For this review, take the finished solid that the model builds, in its own axes (mm). Face numbers are marked on the shaded views. A direction names the side the tool comes from. Round coordinates to 2 decimals unless told otherwise and drop trailing zeros. Write each loop counter-clockwise with the first axis right and the second up, starting at its lowest first coordinate (ties: lowest second). Pieces come first, ordered by that corner, then holes.
from build123d import *

# Parameters (mm, degrees)
F0_W      = 25.4
F0_H      = 69.85
F1_DEPTH  = 12.7
F3_DEPTH  = 12.701
F5_DEPTH  = 19.05
F6_R      = 6.5291939121
F7_DEPTH  = 31.751
F8_W      = 50.8
F8_H      = 31.75
F9_DEPTH  = 6.35
F10_R     = 4.3841328913
F10_R_2   = 4.0648477918
F11_DEPTH = 25.4
F13_DEPTH = 141
F14_R     = 5.08
F15_W     = 12.5349015713
F15_H     = 9.3853002578
F16_DEPTH = 12.7
F18_DEPTH = 25.4
F20_DEPTH = 12.7
F22_DEPTH = 25.4
F24_DEPTH = 25.4


# Not quite as in the source:
# - an extrude ends at something that could not be found from the text; its depth is read off the source's solid
# - a feature names something its author has since deleted; it is built from what else it names


with BuildPart() as f1:
    # F0 (on Front) → F1 (new body)
    with BuildSketch(Plane.XZ):
        with Locations((-34.1177975344, 34.925)):
            Rectangle(F0_W, F0_H)
    extrude(amount=F1_DEPTH)

    # F2 (on face) → F3 (cut, through all)
    with BuildSketch(Plane.XZ.offset(12.7)):
        with BuildLine():
            ThreePointArc((-46.8177975344, 57.1627020836), (-34.8779343498, 69.8199859011), (-21.4177975344, 58.7931149299))
            Line((-21.4177975344, 58.7931149299), (-21.4177975344, 69.85))
            Line((-21.4177975344, 69.85), (-46.8177975344, 69.85))
            Line((-46.8177975344, 69.85), (-46.8177975344, 57.1627020836))
        make_face()
    extrude(amount=-F3_DEPTH, mode=Mode.SUBTRACT)

    # F4 (on face) → F5 (join)
    with BuildSketch(Plane.XZ.offset(12.7)):
        with BuildLine():
            Line((-46.8177975344, 57.1627020836), (-46.8177975344, 54.9187152869))
            ThreePointArc((-46.8177975344, 54.9187152869), (-34.3603071914, 44.1520357407), (-21.4177975344, 54.3305374906))
            Line((-21.4177975344, 54.3305374906), (-21.4177975344, 58.7931149299))
            ThreePointArc((-21.4177975344, 58.7931149299), (-34.8779343498, 69.8199859011), (-46.8177975344, 57.1627020836))
        make_face()
        with BuildLine():
            ThreePointArc((-21.4177975344, 54.3305374906), (-21.194958074, 55.7017298658), (-21.1203918045, 57.0889089552))
            ThreePointArc((-21.1203918045, 57.0889089552), (-35.1496925912, 69.9833496353), (-46.8177975344, 54.9187152869))
            Line((-46.8177975344, 54.9187152869), (-46.8177975344, 57.1627020836))
            ThreePointArc((-46.8177975344, 57.1627020836), (-34.8779343498, 69.8199859011), (-21.4177975344, 58.7931149299))
            Line((-21.4177975344, 58.7931149299), (-21.4177975344, 54.3305374906))
        make_face()
    extrude(amount=F5_DEPTH)

    # F6 (on face) → F7 (cut, through all)
    with BuildSketch(Plane.XZ.offset(31.75)):
        with Locations((-34.0607331136, 57.0889089552)):
            Circle(F6_R)
    extrude(amount=-F7_DEPTH, mode=Mode.SUBTRACT)

    # F8 (on Top) → F9 (join)
    with BuildSketch(Plane.XY):
        with Locations((-35.2321754485, -16.0400984287)):
            Rectangle(F8_W, F8_H)
    extrude(amount=F9_DEPTH)

    # F10 (on face) → F11 (cut)
    with BuildSketch(Plane.XY.offset(6.35)):
        with Locations((-52.9474318027, -24.9871537089)):
            Circle(F10_R)
        with Locations((-18.3323584497, -24.9871537089)):
            Circle(F10_R_2)
    extrude(amount=-F11_DEPTH, mode=Mode.SUBTRACT)

    # F12 (on Front) → F13 (cut, through all)
    with BuildSketch(Plane.XZ):
        with BuildLine():
            ThreePointArc((-47.1297007382, 13.1953000858), (-48.9895726777, 17.6854281464), (-53.4797007382, 19.5453000858))
            ThreePointArc((-53.4797007382, 19.5453000858), (-57.9698287987, 17.6854281464), (-59.8297007382, 13.1953000858))
            ThreePointArc((-59.8297007382, 13.1953000858), (-57.9698287987, 8.7051720253), (-53.4797007382, 6.8453000858))
            ThreePointArc((-53.4797007382, 6.8453000858), (-48.9895726777, 8.7051720253), (-47.1297007382, 13.1953000858))
        make_face()
        with BuildLine():
            ThreePointArc((-59.8297007382, 13.1953000858), (-57.9698287987, 17.6854281464), (-53.4797007382, 19.5453000858))
            Line((-53.4797007382, 19.5453000858), (-59.8297007382, 19.5453000858))
            Line((-59.8297007382, 19.5453000858), (-59.8297007382, 13.1953000858))
        make_face()
        with BuildLine():
            ThreePointArc((-53.4797007382, 6.8453000858), (-57.9698287987, 8.7051720253), (-59.8297007382, 13.1953000858))
            Line((-59.8297007382, 13.1953000858), (-59.8297007382, 6.8453000858))
            Line((-59.8297007382, 6.8453000858), (-53.4797007382, 6.8453000858))
        make_face()
        with BuildLine():
            Line((-47.1297007382, 13.1953000858), (-47.1297007382, 19.5453000858))
            Line((-47.1297007382, 19.5453000858), (-53.4797007382, 19.5453000858))
            ThreePointArc((-53.4797007382, 19.5453000858), (-48.9895726777, 17.6854281464), (-47.1297007382, 13.1953000858))
        make_face()
        with BuildLine():
            ThreePointArc((-8.7253203213, 12.5349001028), (-14.8973108068, 18.7068905883), (-21.0693012923, 12.5349001028))
            ThreePointArc((-21.0693012923, 12.5349001028), (-19.2615671325, 8.170643777), (-14.8973108068, 6.3629096172))
            ThreePointArc((-14.8973108068, 6.3629096172), (-10.533054481, 8.170643777), (-8.7253203213, 12.5349001028))
        make_face()
    extrude(amount=-F13_DEPTH, mode=Mode.SUBTRACT)

    # F14
    f14_edges = [f1.edges().sort_by_distance(p)[0] for p in [
        (-9.832175, -31.915098, 3.175),
        (-60.632175, -31.915098, 3.175),
    ]]
    fillet(f14_edges, radius=F14_R)

    # F15 (on face) → F16 (join)
    with BuildSketch(Plane.YZ.offset(-21.4177975344)):
        with Locations((-6.4325492144, 11.0426501289)):
            Rectangle(F15_W, F15_H)
    extrude(amount=F16_DEPTH)

    # F17 (on face) → F18 (cut)
    with BuildSketch(Plane.XZ.offset(12.7)):
        with BuildLine():
            ThreePointArc((-20.6453823473, 15.7353002578), (-21.221664756, 14.2660198655), (-21.4177975344, 12.7))
            ThreePointArc((-21.4177975344, 12.7), (-19.5579255949, 8.2098719395), (-15.0677975344, 6.35))
            ThreePointArc((-15.0677975344, 6.35), (-10.5776694739, 8.2098719395), (-8.7177975344, 12.7))
            ThreePointArc((-8.7177975344, 12.7), (-8.9139303128, 14.2660198655), (-9.4902127215, 15.7353002578))
            Line((-9.4902127215, 15.7353002578), (-20.6453823473, 15.7353002578))
        make_face()
        with BuildLine():
            ThreePointArc((-9.4902127215, 15.7353002578), (-15.0677975344, 19.05), (-20.6453823473, 15.7353002578))
            Line((-20.6453823473, 15.7353002578), (-9.4902127215, 15.7353002578))
        make_face()
        with BuildLine():
            ThreePointArc((-8.7177975344, 12.7), (-10.5776694739, 8.2098719395), (-15.0677975344, 6.35))
            Line((-15.0677975344, 6.35), (-9.8321754485, 6.35))
            Line((-9.8321754485, 6.35), (-8.7177975344, 6.35))
            Line((-8.7177975344, 6.35), (-8.7177975344, 12.7))
        make_face()
        with BuildLine():
            Line((-8.7177975344, 15.7353002578), (-9.4902127215, 15.7353002578))
            ThreePointArc((-9.4902127215, 15.7353002578), (-8.9139303128, 14.2660198655), (-8.7177975344, 12.7))
            Line((-8.7177975344, 12.7), (-8.7177975344, 15.7353002578))
        make_face()
    extrude(amount=-F18_DEPTH, mode=Mode.SUBTRACT)

    # F19 (on face) → F20 (join)
    with BuildSketch(Plane(origin=(-46.8177975344, 0, 0), x_dir=(0, -1, 0), z_dir=(-1, 0, 0))):
        Polygon((12.7, 16.4465010166), (0, 16.4465010166), (0, 6.35), (0.1650984287, 6.35), (12.7, 6.35), align=None)
    extrude(amount=F20_DEPTH)

    # F21 (on face) → F22 (cut)
    with BuildSketch(Plane.XZ.offset(12.7)):
        with BuildLine():
            Line((-59.5177975344, 6.35), (-53.1677975344, 6.35))
            ThreePointArc((-53.1677975344, 6.35), (-57.6579255949, 8.2098719395), (-59.5177975344, 12.7))
            Line((-59.5177975344, 12.7), (-59.5177975344, 6.35))
        make_face()
        with BuildLine():
            Line((-21.4177975344, 15.7353002578), (-21.4177975344, 12.7))
            ThreePointArc((-21.4177975344, 12.7), (-21.221664756, 14.2660198655), (-20.6453823473, 15.7353002578))
            Line((-20.6453823473, 15.7353002578), (-21.4177975344, 15.7353002578))
        make_face()
        with BuildLine():
            ThreePointArc((-59.5177975344, 12.7), (-59.204311952, 14.6705313207), (-58.2948073971, 16.4465010166))
            Line((-58.2948073971, 16.4465010166), (-59.5177975344, 16.4465010166))
            Line((-59.5177975344, 16.4465010166), (-59.5177975344, 12.7))
        make_face()
        with BuildLine():
            Line((-58.2948073971, 16.4465010166), (-48.0407876717, 16.4465010166))
            ThreePointArc((-48.0407876717, 16.4465010166), (-53.1677975344, 19.05), (-58.2948073971, 16.4465010166))
        make_face()
        with BuildLine():
            ThreePointArc((-53.1677975344, 6.35), (-48.6776694739, 8.2098719395), (-46.8177975344, 12.7))
            ThreePointArc((-46.8177975344, 12.7), (-47.1312831168, 14.6705313207), (-48.0407876717, 16.4465010166))
            Line((-48.0407876717, 16.4465010166), (-58.2948073971, 16.4465010166))
            ThreePointArc((-58.2948073971, 16.4465010166), (-59.204311952, 14.6705313207), (-59.5177975344, 12.7))
            ThreePointArc((-59.5177975344, 12.7), (-57.6579255949, 8.2098719395), (-53.1677975344, 6.35))
        make_face()
    extrude(amount=-F22_DEPTH, mode=Mode.SUBTRACT)

    # F23 (on face) → F24 (cut)
    with BuildSketch(Plane.XZ.offset(12.7)):
        with BuildLine():
            Line((-46.8177975344, 12.7), (-46.8177975344, 16.4465010166))
            Line((-46.8177975344, 16.4465010166), (-48.0407876717, 16.4465010166))
            ThreePointArc((-48.0407876717, 16.4465010166), (-47.1312831168, 14.6705313207), (-46.8177975344, 12.7))
        make_face()
    extrude(amount=-F24_DEPTH, mode=Mode.SUBTRACT)


solid = f1.part
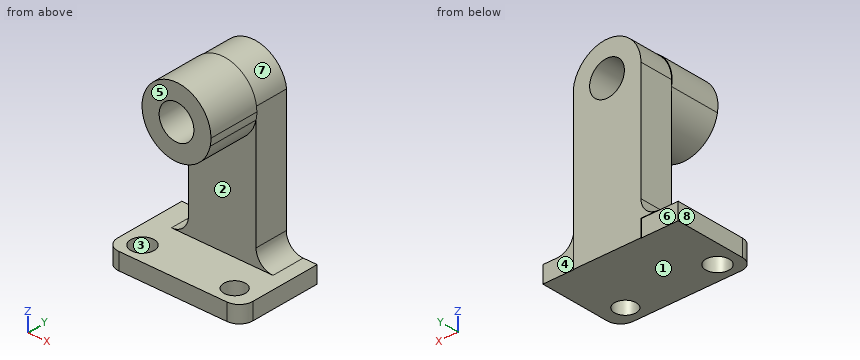
(1) We need section A-A, the plane y = -19. Give the boundary of the cut face in (x, z).
Geometry check:
outline: (-60.63, 0) - (-9.83, 0) - (-9.83, 6.35) - (-60.63, 6.35) - close; circle Ø25.88 at (-34.06, 57.09); hole circle Ø13.06 at (-34.06, 57.09)
(2) Mouldability with a two-part tool opening along Y and no side actions: class the marked faces 1, 2, 3 and 4 as pulls with the +Y half, pulls with the -Y half, needs draft (parallel to the pull), parting line crosses it, or undercut.
Geometry check:
face 1: needs draft
face 2: pulls with the -Y half
face 3: undercut
face 4: pulls with the +Y half
(3) For the marked faces 5, 6, 7 and 8, list the 3-axis set-ups (+Z, -Z, +X, -X, +Y, -Y) from which the entire face can be reached by the end or side of a thin tool; tool diameter is ignored.
Geometry check:
face 5: +Z, +X, -X, -Y
face 6: -Z, -X, +Y
face 7: +Z, +Y
face 8: +Z, -Z, -X, +Y, -Y
(4) We need section B-B, the plane y = -28. Give the boundary of the cut face in (x, z), and give its area (3 significant figures).
Geometry check:
outline: (-60.5, 0) - (-56.13, 0) - (-56.13, 6.35) - (-60.5, 6.35) - close; (-49.76, 0) - (-21.06, 0) - (-21.06, 6.35) - (-49.76, 6.35) - close; circle Ø25.88 at (-34.06, 57.09); (-15.6, 0) - (-9.97, 0) - (-9.97, 6.35) - (-15.6, 6.35) - close; hole circle Ø13.06 at (-34.06, 57.09)
area: 638 mm2
(5) We need section D-D, the plane z = 61.5. Give the boundary of the cut face in (x, y).
Geometry check:
outline: (-46.23, -31.75) - (-38.87, -31.75) - (-38.87, 0) - (-46.03, 0) - (-46.03, -12.7) - (-46.23, -12.7) - close; (-29.25, -31.75) - (-21.9, -31.75) - (-21.9, -12.7) - (-22.09, -12.7) - (-22.09, 0) - (-29.25, 0) - close
(6) For pin 1 Ø5 at (x, z) = (-43.5, 30.5) entering from -Y; pin 2 Ø17 at (x, z) = (-34.06, 57.09) entering from -Y; pin 3 Ø3 at (x, z) = (-56, 4.5) entering from +Y, all flat-tipped, find the tip position at first contact; note any pin that passes through.
Geometry check:
pin 1: stops at y = -12.7
pin 2: stops at y = -31.75
pin 3: stops at y = -0.17
(7) We need section C-C, the plane y = -4.5. Give the boundary of the cut face in (x, z).
Geometry check:
outline: (-60.63, 0) - (-9.83, 0) - (-9.83, 6.35) - (-15.07, 6.35) arc R6.35 cw to (-21.42, 12.7) - (-21.42, 58.79) arc R12.76 ccw to (-46.82, 57.16) - (-46.82, 12.7) arc R6.35 cw to (-53.17, 6.35) - (-60.63, 6.35) - close; hole circle Ø13.06 at (-34.06, 57.09)
(8) For line 1 along Z through (x, y) = (-32, -30); line 2 along Z through (x, y) = (-17, -19); line 3 along Y through (x, z) = (-38, 10), list the stretches that pass through material, from the lowest coordinate up.
Geometry check:
line 1: z = 0 to 6.35, 44.31 to 50.89, 63.28 to 69.86
line 2: z = 0 to 6.35
line 3: y = -12.7 to 0
